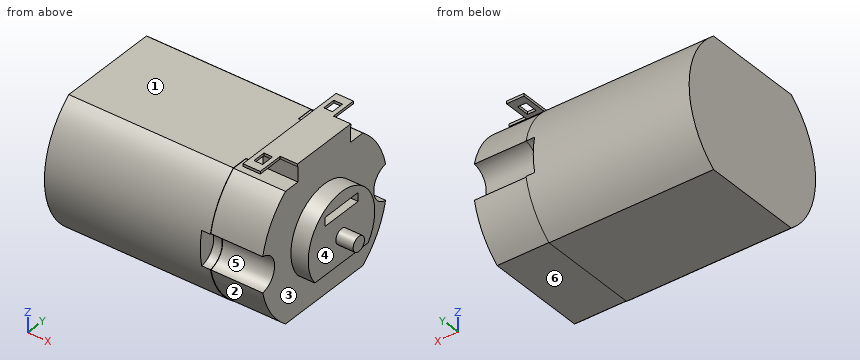
```python
from build123d import *

# Parameters (mm, degrees)
BOSS_EXTRUDE1_DEPTH = 25
SKETCH2_R           = 2
CUT_EXTRUDE1_DEPTH  = 7
SKETCH3_W           = 1
SKETCH3_H           = 5
BOSS_EXTRUDE2_DEPTH = 2
SKETCH4_R           = 0.85
BOSS_EXTRUDE3_DEPTH = 2
SKETCH5_W           = 4
SKETCH5_H           = 8
BOSS_EXTRUDE4_DEPTH = 2
SKETCH6_W           = 2
SKETCH6_H           = 0.3
BOSS_EXTRUDE5_DEPTH = 3
SKETCH7_W           = 1
SKETCH7_H           = 1.5
CUT_EXTRUDE2_DEPTH  = 1
CUT_EXTRUDE3_START  = -6
CUT_EXTRUDE3_DEPTH  = 6


with BuildPart() as part:
    # Sketch1 → Boss-Extrude1 (new body)
    with BuildSketch(Plane(origin=(0, 0, 0), x_dir=(0, 0, -1), z_dir=(1, 0, 0))):
        with BuildLine():
            Line((-7.5, 5.830951895), (-7.5, -5.830951895))
            ThreePointArc((-7.5, -5.830951895), (0, -9.5), (7.5, -5.830951895))
            Line((7.5, -5.830951895), (7.5, 5.830951895))
            ThreePointArc((7.5, 5.830951895), (0, 9.5), (-7.5, 5.830951895))
        make_face()
    extrude(amount=BOSS_EXTRUDE1_DEPTH)

    # Sketch2 → Cut-Extrude1 (cut)
    with BuildSketch(Plane(origin=(25, 0, 0), x_dir=(0, 0, -1), z_dir=(1, 0, 0))):
        with Locations((0, 9.5)):
            Circle(SKETCH2_R)
        with Locations((0, -9.5)):
            Circle(SKETCH2_R)
    extrude(amount=-CUT_EXTRUDE1_DEPTH, mode=Mode.SUBTRACT)

    # Sketch3 → Boss-Extrude2 (add)
    with BuildSketch(Plane(origin=(25, 0, 0), x_dir=(0, 0, -1), z_dir=(1, 0, 0))):
        with BuildLine():
            Line((3, 4), (3, -4))
            ThreePointArc((3, -4), (-5, 0), (3, 4))
        make_face()
        with Locations((-3, 0)):
            Rectangle(SKETCH3_W, SKETCH3_H, mode=Mode.SUBTRACT)
    extrude(amount=BOSS_EXTRUDE2_DEPTH)

    # Sketch4 → Boss-Extrude3 (add)
    with BuildSketch(Plane(origin=(27, 0, 0), x_dir=(0, 0, -1), z_dir=(1, 0, 0))):
        Circle(SKETCH4_R)
    extrude(amount=BOSS_EXTRUDE3_DEPTH)

    # Sketch5 → Boss-Extrude4 (add)
    with BuildSketch(Plane.XY.offset(7.5)):
        with Locations((23, 0)):
            Rectangle(SKETCH5_W, SKETCH5_H)
    extrude(amount=BOSS_EXTRUDE4_DEPTH)

    # Sketch6 → Boss-Extrude5 (add)
    with BuildSketch(Plane.XZ.offset(4)):
        with Locations((22, 9.35)):
            Rectangle(SKETCH6_W, SKETCH6_H)
    boss_extrude5 = extrude(amount=BOSS_EXTRUDE5_DEPTH)

    # Mirror1: Boss-Extrude5 across plane
    add(boss_extrude5.mirror(Plane.ZX))

    # Sketch7 → Cut-Extrude2 (cut)
    with BuildSketch(Plane.XY.offset(9.5)):
        with Locations((22, -5.25)):
            Rectangle(SKETCH7_W, SKETCH7_H)
        with Locations((22, 5.25)):
            Rectangle(SKETCH7_W, SKETCH7_H)
    extrude(amount=-CUT_EXTRUDE2_DEPTH, mode=Mode.SUBTRACT)

    # Sketch8 → Cut-Extrude3 (cut)
    with BuildSketch(Plane(origin=(25, 0, 0), x_dir=(0, 0, -1), z_dir=(1, 0, 0)).offset(CUT_EXTRUDE3_START)):
        with BuildLine():
            Line((-7.45, 5.813776741), (-7.45, 3.95))
            Line((-7.45, 3.95), (-9.2, 3.95))
            Line((-9.2, 3.95), (-9.2, 4))
            Line((-9.2, 4), (-7.5, 4))
            Line((-7.5, 4), (-7.5, 5.830951895))
            ThreePointArc((-7.5, 5.830951895), (-5.049761967, 8.04673251), (-1.988888803, 9.289473684))
            ThreePointArc((-1.988888803, 9.289473684), (0, 7.5), (1.988888803, 9.289473684))
            ThreePointArc((1.988888803, 9.289473684), (5.049761967, 8.04673251), (7.5, 5.830951895))
            Line((7.5, 5.830951895), (7.5, -5.830951895))
            ThreePointArc((7.5, -5.830951895), (5.049761967, -8.04673251), (1.988888803, -9.289473684))
            ThreePointArc((1.988888803, -9.289473684), (0, -7.5), (-1.988888803, -9.289473684))
            ThreePointArc((-1.988888803, -9.289473684), (-5.049761967, -8.04673251), (-7.5, -5.830951895))
            Line((-7.5, -5.830951895), (-7.5, -4))
            Line((-7.5, -4), (-9.2, -4))
            Line((-9.2, -4), (-9.2, -3.95))
            Line((-9.2, -3.95), (-7.45, -3.95))
            Line((-7.45, -3.95), (-7.45, -5.813776741))
            ThreePointArc((-7.45, -5.813776741), (-5.039140418, -7.994345742), (-2.032001592, -9.228947368))
            ThreePointArc((-2.032001592, -9.228947368), (0, -7.45), (2.032001592, -9.228947368))
            ThreePointArc((2.032001592, -9.228947368), (5.039140418, -7.994345742), (7.45, -5.813776741))
            Line((7.45, -5.813776741), (7.45, 5.813776741))
            ThreePointArc((7.45, 5.813776741), (5.039140418, 7.994345742), (2.032001592, 9.228947368))
            ThreePointArc((2.032001592, 9.228947368), (0, 7.45), (-2.032001592, 9.228947368))
            ThreePointArc((-2.032001592, 9.228947368), (-5.039140418, 7.994345742), (-7.45, 5.813776741))
        make_face()
    extrude(amount=CUT_EXTRUDE3_DEPTH, mode=Mode.SUBTRACT)


solid = part.part
```
Geometry check sheet. Reference: the model listing, model coordinates, mm. Face numbers are marked on the shaded views. A direction names the side the tool comes from. Round coordinates to 2 decimals unless told otherwise and drop trailing zeros. Loops run counter-clockwise (first coordinate to the right, second up) from the corner with the lowest first, then second, coordinate; pieces in that order, holes last. Notation, with made-up numbers: (16.5, 65.25) - (72.5, 65.25) arc R9 cw to (72.5, 73.25) - close; hole circle Ø5 at (6, 65.25). An arc over 180 degrees is marked (long way). Write item = value, one per line. Start each with the question number.
1. Section check B-B on y = 0. Enter the section's corners in (x, z).
2. Section check D-D on z = -6. Enter the section's corners in (x, y), then the cut area to 3 significant figures.
3. Section check A-A on x = 20. Enter the section's corners in (y, z).
4. Mould release check, pull along Z, two halves, no side actions. Record for the marked faces 4, 5 and 6: released by +Z, released by -Z, zero draft, split by the parting line, or undercut.
5. Set-up check for the marked faces 1, 2 and 3: record each of +Z, -Z, +X, -X, +Y, -Y from which the full face is reachable in a straight line by a thin tool's end or side.
6. Section check C-C on z = 0. Enter the section's corners in (x, y).
7. Thickness scan on line 1 (Z direction, x = 1.75, y = -0.75); line 2 (X direction, y = 3.25, z = -2.25); line 3 (X direction, y = -3.25, z = 5.75). Record the ranges inside material, lowest first.
8. Depth check by flat-ended pin: pin 1 (4 mm diameter, centred on x = 17, y = 2, fed in from +Z); pin 2 (1.5 mm diameter, centred on x = 15.5, z = -2, fed in from +Y); pin 3 (1.6 mm diameter, centred on y = -1, z = 8.5, fed in from -X). Enter the tip coordinate at first touch or a pass-through.
Working result:
q1.outline = (0, -7.5) - (19, -7.5) - (19, -7.45) - (25, -7.45) - (25, -3) - (27, -3) - (27, -0.85) - (29, -0.85) - (29, 0.85) - (27, 0.85) - (27, 2.5) - (25, 2.5) - (25, 3.5) - (27, 3.5) - (27, 5) - (25, 5) - (25, 9.5) - (21, 9.5) - (21, 7.5) - (0, 7.5) - close
q2.outline = (0, -7.37) - (19, -7.37) - (19, -7.3) - (25, -7.3) - (25, 7.3) - (19, 7.3) - (19, 7.37) - (0, 7.37) - close
q2.area = 367 mm^2
q3.outline = (-9.23, -2.03) arc R9.45 ccw to (-5.81, -7.45) - (5.81, -7.45) arc R9.45 ccw to (9.23, -2.03) arc R2.05 cw to (9.23, 2.03) arc R9.45 ccw to (5.81, 7.45) - (3.95, 7.45) - (3.95, 7.5) - (-3.95, 7.5) - (-3.95, 7.45) - (-5.81, 7.45) arc R9.45 ccw to (-9.23, 2.03) arc R2.05 cw to start
q4.face_4 = zero draft
q4.face_5 = undercut
q4.face_6 = released by -Z
q5.face_1 = +Z, -X, +Y, -Y
q5.face_2 = -Z, +X, -Y
q5.face_3 = +X
q6.outline = (0, -9.5) - (18, -9.5) - (18, -7.5) - (19, -7.5) - (19, -7.45) - (25, -7.45) - (25, -5) - (27, -5) - (27, -0.85) - (29, -0.85) - (29, 0.85) - (27, 0.85) - (27, 5) - (25, 5) - (25, 7.45) - (19, 7.45) - (19, 7.5) - (18, 7.5) - (18, 9.5) - (0, 9.5) - close
q7.line_1 = -7.5 to 7.5
q7.line_2 = 0 to 27
q7.line_3 = 0 to 25
q8.pin_1 = 7.5
q8.pin_2 = 9.42
q8.pin_3 = 21
